Autodesk Inventor part; units mm, degrees
ref_plane "to_bearing_XY" through (0, 79, -8.5) normal (0, 0, 1) x (1, 0, 0)
ref_plane "to_bearing_YZ" through (0, 79, -8.5) normal (1, 0, 0) x (0, 1, 0)
ref_plane "to_bearing_ZX" through (0, 79, -8.5) normal (0, 1, 0) x (0, 0, 1)
sketch "Sketch_7" plane through (0, 0, 0) normal (0, 0, 1) x (1, 0, 0)
  line L0 (-32.5, 79) -> (-32.5, 0)
  line L1 (-32.5, 0) -> (32.5, 0)
  line L2 (32.5, 0) -> (32.5, 79)
  arc A0 (32.5, 79) -> (-32.5, 79) centre (0, 79) ccw
extrude "Extrusion1" add sketch "Sketch_7" against normal blind 19
sketch "Sketch_8" plane through (0, 0, 0) normal (1, 0, 0) x (0, 0, -1)
  line L0 (19, 79) -> (2, 79)
  line L1 (2, 79) -> (2, 106.5)
  line L2 (2, 106.5) -> (15, 106.5)
  line L3 (15, 106.5) -> (15, 108)
  line L4 (15, 108) -> (17, 108)
  line L5 (17, 108) -> (17, 106.5)
  line L6 (17, 106.5) -> (19, 106.5)
  line L7 (19, 106.5) -> (19, 79)
  line L8 (19, 79) -> (2, 79)
revolve "Revolution1" cut sketch "Sketch_8" angle 360 about axis through (0, 79, -19) along (0, 0, -1)
sketch "Sketch_1" plane through (0, 0, 0) normal (1, 0, 0) x (0, 0, -1)
  line L0 (19, 79) -> (0, 79)
  line L1 (0, 79) -> (0, 103)
  line L2 (0, 103) -> (19, 103)
  line L3 (19, 103) -> (19, 79)
  line L4 (19, 79) -> (0, 79)
revolve "Revolution2" cut sketch "Sketch_1" angle 360 about axis through (0, 79, -19) along (0, 0, -1)
sketch "Sketch4" plane through (0, 0, -19) normal (0, 0, -1) x (-1, 0, 0)
  point P0 (13, 13)
hole "Hole1" at (-13, 13, -19) direction (0, 0, 1) diameter 12 depth 19
pattern_linear "Rectangular Pattern1" count 2 spacing 26 along (1, 0, 0) count 2 spacing 26 along (0, 1, 0) of "Hole1"
ref_plane "to_bearing_XY" through (0, 79, -8.5) normal (0, 0, 1) x (1, 0, 0)
ref_plane "to_bearing_YZ" through (0, 79, -8.5) normal (1, 0, 0) x (0, 1, 0)
ref_plane "to_bearing_ZX" through (0, 79, -8.5) normal (0, 1, 0) x (0, 0, 1)
ref_plane "to_retaining_ring_XY" through (0, 79, -17) normal (0, 0, -1) x (1, 0, 0)
ref_plane "to_retaining_ring_YZ" through (0, 79, -17) normal (1, 0, 0) x (0, -1, 0)
ref_plane "to_retaining_ring_ZX" through (0, 79, -17) normal (0, -1, 0) x (0, 0, -1)
properties part number "SBGSMA6006ZZ-40_h"
Geometry: final body of the model. Coordinates: model frame, mm. A direction names the side the tool comes from. Coordinates: 2 decimals unless noted, no trailing zeros. Order: outer loops, then holes, each group sorted by start corner. A loop starts at its lowest first (then second) coordinate and runs counter-clockwise, first axis right, second up. Notation, with made-up numbers: M -1,40 L 22,40 A8 cw 22,45 Z; hole C -11.5,-6.75 d1. An arc over 180 degrees is marked long. Answer in a Markdown table with one row per item. Add a question column.
Q1. Section query C-C on z = -5.5. Return the cut outline in (x, y).
Q2. Section query A-A on y = 39. Return the cut outline in (x, z).
Q3. Section query B-B on x = 0. Return the cut outline in (y, z), and give its area (3 significant figures).
Q4. Contact query for flat-ended pins moving along their axis: P1, Ø1, axis at x = 20, z = -11.5, coming from the +Y side; P2, Ø2, axis at x = 9, z = -6.5, coming from the +Y side; P3, Ø8, axis at x = 20.5, z = -16.5, coming from the +Y side. Output: stop coordinate, or through.
Q5. Mould query, pull axis Z, two halves, no side actions, for faces 1 (the flat face through (22, 96, -17)), 2 (the flat face through (0, 44, -19)), 3 (the cylindrical face through (0.715, 111.492, -9.367)). Classes: released by +Z, released by -Z, zero draft, split by the parting line, or undercut.
Q6. Reachability of faces 4 (the cylindrical face through (1.209, 51.527, -18.014)), 5 (the cylindrical face through (8.71, 106.66, -16.01)), 6 (the flat face through (-32.5, 40, -9)) from +Z, -Z, +X, -X, +Y, -Y: full face, straight path, thin tool, end or side. Return the list, or none.
Q7. Line query: L1, parallel to X at y = 13, z = -8; L2, parallel to Z at x = -25, y = 66.5; L3, parallel to Y at x = -9, z = -16.5. Output: solid intervals per line, ascending.
Q8. Section query D-D on x = 13. Return the cut outline in (y, z).
Completed:
| question | item | result |
|---|---|---|
| 1 | outline | M -32.5,0 L 32.5,0 L 32.5,79 A32.5 ccw -32.5,79 Z; hole C 0,79 d55; hole C -13,13 d12; hole C -13,39 d12; hole C 13,13 d12; hole C 13,39 d12 |
| 2 | outline | M -32.5,-19 L -19,-19 L -19,0 L -32.5,0 Z; M -7,-19 L 7,-19 L 7,0 L -7,0 Z; M 19,-19 L 32.5,-19 L 32.5,0 L 19,0 Z |
| 3 | outline | M 0,-19 L 51.5,-19 L 51.5,-17 L 50,-17 L 50,-15 L 51.5,-15 L 51.5,-2 L 55,-2 L 55,0 L 0,0 Z; M 103,-2 L 106.5,-2 L 106.5,-15 L 108,-15 L 108,-17 L 106.5,-17 L 106.5,-19 L 111.5,-19 L 111.5,0 L 103,0 Z |
| 3 | area | 1,080 mm2 |
| 4 | P1 | stops at y = 105 |
| 4 | P2 | stops at y = 110.5 |
| 4 | P3 | stops at y = 107 |
| 5 | face 1 | undercut |
| 5 | face 2 | released by -Z |
| 5 | face 3 | zero draft |
| 6 | face 4 | -Z |
| 6 | face 5 | none |
| 6 | face 6 | +Z, -Z, -X, +Y, -Y |
| 7 | L1 | x = -32.5 to -19, -7 to 7, 19 to 32.5 |
| 7 | L2 | z = -19 to -17, -15 to 0 |
| 7 | L3 | y = 0 to 8.53, 17.47 to 34.53, 43.47 to 51.43, 106.57 to 110.23 |
| 8 | outline | M 0,-19 L 7,-19 L 7,0 L 0,0 Z; M 19,-19 L 33,-19 L 33,0 L 19,0 Z; M 45,-19 L 54.77,-19 L 54.77,-17 L 53.08,-17 L 53.08,-15 L 54.77,-15 L 54.77,-2 L 58.83,-2 L 58.83,0 L 45,0 Z; M 99.17,-2 L 103.23,-2 L 103.23,-15 L 104.92,-15 L 104.92,-17 L 103.23,-17 L 103.23,-19 L 108.79,-19 L 108.79,0 L 99.17,0 Z |
